The listing builds one solid part. Answer for the finished solid, in the listing's coordinates (mm). Face numbers are marked on the shaded views. A direction names the side the tool comes from. Give positions to 0.01 mm unless a question says otherwise; leave off trailing zeros. Write each loop counter-clockwise with the first axis right and the second up, starting at its lowest first coordinate (ties: lowest second). Pieces come first, ordered by that corner, then holes. Notation, with made-up numbers: (15, 74) -> (19, 74) arc R21 cw to (19, 101) -> close; hole circle Ø9 at (-16.75, 11). An arc over 180 degrees is marked (long way). Put each result on its own line as item: value. Start each with the question number.
1) For a pull along Y with two mould halves and no side action, classify the marked faces 1, 2 and 3 as released by +Y, released by -Y, zero draft, split by the parting line, or undercut.
2) A cutting plane is placed at D-D (z = 5.75). Write down the section's boundary in (x, y) (3 decimals), then the cut area to 3 significant figures.
3) A cutting plane is placed at B-B (y = 0). Write down the section's boundary in (x, z) (3 decimals).
4) For the marked faces 4, 5 and 6, determine the directions among +Z, -Z, +X, -X, +Y, -Y from which every point of the face is accessible in a straight line to the end or side of a thin tool.
5) A cutting plane is placed at C-C (x = -3). Write down the section's boundary in (y, z).
6) A cutting plane is placed at A-A (z = 2.5). Write down the section's boundary in (x, y) (3 decimals).
7) Find the intervals of material crossed by line 1 along Y through (x, z) = (9, 1.75); line 2 along X through (y, z) = (-1.5, 5.5); line 3 along X through (y, z) = (1.25, 4.75), in increasing order. Write a range as from..to.
8) Flat-ended cylindrical pins translate along their axes: pin 1 Ø1.6 at (x, y) = (-17.5, 1) entering from +Z; pin 2 Ø1.2 at (x, y) = (-2.5, 4.5) entering from -Z; pin 3 Ø4 at (y, z) = (-6, 5) entering from -X. Find the tip coordinate at first contact, or state that the pin passes through.
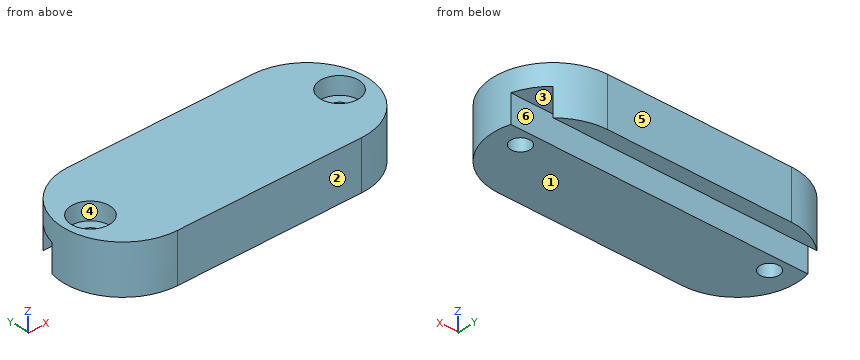
from build123d import *

# Parameters (mm, degrees)
BOSS_EXTRUDE1_DEPTH     = 7
SKETCH3_W               = 8
SKETCH3_H               = 4
CUT_EXTRUDE1_DEPTH      = 6.459407384
CUT_EXTRUDE1_DEPTH_BACK = 39.259407384
SKETCH6_R               = 1.4
CUT_EXTRUDE3_DEPTH      = 1
CUT_EXTRUDE3_DEPTH_BACK = 8
SKETCH8_R               = 2.75
CUT_EXTRUDE4_DEPTH      = 1
CUT_EXTRUDE4_DEPTH_BACK = 2.5


with BuildPart() as part:
    # Sketch1 → Boss-Extrude1 (new body)
    with BuildSketch(Plane.XY):
        with BuildLine():
            Line((-13.359407384, -8.5), (13.359407384, -8.5))
            ThreePointArc((13.359407384, -8.5), (21.859407384, 0), (13.359407384, 8.5))
            Line((13.359407384, 8.5), (-13.359407384, 8.5))
            ThreePointArc((-13.359407384, 8.5), (-21.859407384, 0), (-13.359407384, -8.5))
        make_face()
    extrude(amount=BOSS_EXTRUDE1_DEPTH)

    # Sketch3 → Cut-Extrude1 (cut, two sides)
    with BuildSketch(Plane(origin=(16.4, 0, 0), x_dir=(0, 0, -1), z_dir=(1, 0, 0))) as cut_extrude1_sk:
        with Locations((0, 4.247574753)):
            Rectangle(SKETCH3_W, SKETCH3_H)
    extrude(amount=CUT_EXTRUDE1_DEPTH, mode=Mode.SUBTRACT)
    extrude(cut_extrude1_sk.sketch, amount=-CUT_EXTRUDE1_DEPTH_BACK, mode=Mode.SUBTRACT)

    # Sketch6 → Cut-Extrude3 (cut, two sides)
    with BuildSketch(Plane(origin=(0, 0, 0), x_dir=(-1, 0, 0), z_dir=(0, 0, -1))) as cut_extrude3_sk:
        with Locations((-18.075, 0)):
            Circle(SKETCH6_R)
        with Locations((18.075, 0)):
            Circle(SKETCH6_R)
    extrude(amount=CUT_EXTRUDE3_DEPTH, mode=Mode.SUBTRACT)
    extrude(cut_extrude3_sk.sketch, amount=-CUT_EXTRUDE3_DEPTH_BACK, mode=Mode.SUBTRACT)

    # Sketch8 → Cut-Extrude4 (cut, two sides)
    with BuildSketch(Plane.XY.offset(7)) as cut_extrude4_sk:
        with Locations((-18.075, 0)):
            Circle(SKETCH8_R)
        with Locations((18.075, 0)):
            Circle(SKETCH8_R)
    extrude(amount=CUT_EXTRUDE4_DEPTH, mode=Mode.SUBTRACT)
    extrude(cut_extrude4_sk.sketch, amount=-CUT_EXTRUDE4_DEPTH_BACK, mode=Mode.SUBTRACT)


solid = part.part
Reply:
1. face 1: zero draft
1. face 2: released by -Y
1. face 3: undercut
2. outline: (-13.359, -8.5) -> (13.359, -8.5) arc R8.5 ccw to (13.359, 8.5) -> (-13.359, 8.5) arc R8.5 ccw to start; hole circle Ø5.5 at (-18.075, 0); hole circle Ø5.5 at (18.075, 0)
2. area: 634 mm2
3. outline: (-21.859, 0) -> (-19.475, 0) -> (-19.475, 4.5) -> (-20.825, 4.5) -> (-20.825, 7) -> (-21.859, 7) -> close; (-16.675, 0) -> (16.675, 0) -> (16.675, 4.5) -> (15.325, 4.5) -> (15.325, 7) -> (-15.325, 7) -> (-15.325, 4.5) -> (-16.675, 4.5) -> close; (19.475, 0) -> (21.859, 0) -> (21.859, 7) -> (20.825, 7) -> (20.825, 4.5) -> (19.475, 4.5) -> close
4. face 4: +Z
4. face 5: +Z, -Z, +X, -X, +Y
4. face 6: -Z, +X, -X
5. outline: (-8.5, 0) -> (2.25, 0) -> (2.25, 4) -> (6.25, 4) -> (6.25, 0) -> (8.5, 0) -> (8.5, 7) -> (-8.5, 7) -> close
6. outline: (-21.557, 2.248) arc R8.5 ccw to (-13.359, -8.5) -> (13.359, -8.5) arc R8.5 ccw to (21.557, 2.248) -> close; (-19.123, 6.248) -> (19.123, 6.248) arc R8.5 ccw to (13.359, 8.5) -> (-13.359, 8.5) arc R8.5 ccw to start; hole circle Ø2.8 at (-18.075, 0); hole circle Ø2.8 at (18.075, 0)
7. line 1: y = -8.5..2.25, 6.25..8.5
7. line 2: x = -21.73..-20.38, -15.77..15.77, 20.38..21.73
7. line 3: x = -21.77..-20.52, -15.63..15.63, 20.52..21.77
8. pin 1: stops at z = 4.5
8. pin 2: stops at z = 4
8. pin 3: stops at x = -20.86
